Input: part model. Units: mm. Frame: model coordinates. Face numbers are marked on the shaded views. A direction names the side the tool comes from. Give positions to 0.01 mm unless a question says otherwise; leave off trailing zeros. Loops run counter-clockwise (first coordinate to the right, second up) from the corner with the lowest first, then second, coordinate; pieces in that order, holes last. Notation, with made-up numbers: (20, 50) - (52, 50) arc R13 cw to (52, 58) - close; hole circle Ø7 at (59.5, -36). An arc over 180 degrees is marked (long way). Answer as a JSON object with one key per item and string values.
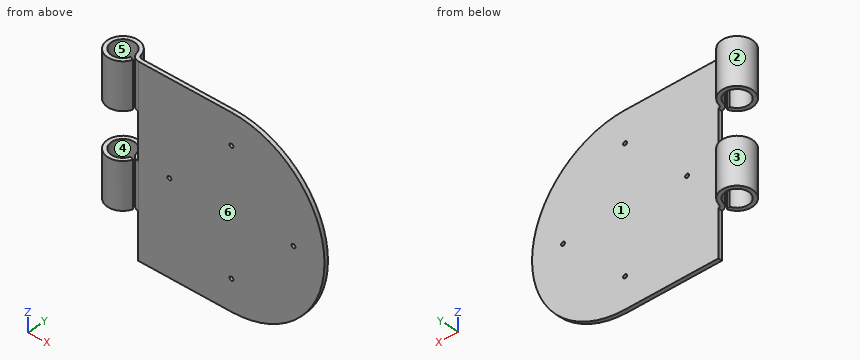
from build123d import *

# Parameters (mm, degrees)
BOSS_EXTRUDE1_DEPTH     = 76.2
CUT_EXTRUDE1_DEPTH      = 109.055004078
CUT_EXTRUDE1_DEPTH_BACK = 109.055004078
SKETCH2_W               = 19.05
SKETCH2_H               = 13.97
SKETCH3_R               = 0.79375
CUT_EXTRUDE2_DEPTH      = 114.673225775


with BuildPart() as part:
    # Sketch1 → Boss-Extrude1 (new body)
    with BuildSketch(Plane.XY):
        with BuildLine():
            Line((6.006670832, -2.059710057), (4.505003124, -1.544782543))
            ThreePointArc((4.505003124, -1.544782543), (-4.752599731, 0.306923518), (4.66627796, 0.9525))
            ThreePointArc((4.66627796, 0.9525), (5.769083619, -0.871844425), (7.777129933, -1.5875))
            Line((7.777129933, -1.5875), (83.977129933, -1.5875))
            Line((83.977129933, -1.5875), (83.977129933, 0))
            Line((83.977129933, 0), (7.777129933, 0))
            ThreePointArc((7.777129933, 0), (6.773106776, 0.357827788), (6.221703947, 1.27))
            ThreePointArc((6.221703947, 1.27), (-6.336799641, 0.409231357), (6.006670832, -2.059710057))
        make_face()
    extrude(amount=BOSS_EXTRUDE1_DEPTH)

    # Sketch2 → Cut-Extrude1 (cut, two sides: drawn at the far end of the back side and taken through both)
    with BuildSketch(Plane(origin=(69.85, -1.5875, 0), x_dir=(0, 0, -1), z_dir=(0, 1, 0)).offset(-CUT_EXTRUDE1_DEPTH_BACK)):
        with Locations((-9.525, 69.215)):
            Rectangle(SKETCH2_W, SKETCH2_H)
        with Locations((-47.625, 69.215)):
            Rectangle(SKETCH2_W, SKETCH2_H)
    extrude(amount=CUT_EXTRUDE1_DEPTH + CUT_EXTRUDE1_DEPTH_BACK, mode=Mode.SUBTRACT)

    # Sketch3 → Cut-Extrude2 (cut, through all)
    with BuildSketch(Plane(origin=(0, -1.5875, 0), x_dir=(1, 0, 0), z_dir=(0, 1, 0))):
        with BuildLine():
            Line((83.977129933, 0), (45.877129933, 0))
            ThreePointArc((45.877129933, 0), (72.817898258, -11.159231598), (83.977129933, -38.09999989))
            Line((83.977129933, -38.09999989), (83.977129933, 0))
        make_face()
        with BuildLine():
            Line((83.977129933, -76.2), (83.977129933, -38.09999989))
            ThreePointArc((83.977129933, -38.09999989), (72.817898336, -65.040768324), (45.877129933, -76.2))
            Line((45.877129933, -76.2), (83.977129933, -76.2))
        make_face()
        with Locations(Location((45.877129933, -63.5, 0), (0, 0, 90))):
            Circle(SKETCH3_R)
        with Locations(Location((20.477129933, -38.1, 0), (0, 0, 90))):
            Circle(SKETCH3_R)
        with Locations(Location((71.277129933, -38.1, 0), (0, 0, 90))):
            Circle(SKETCH3_R)
        with Locations(Location((45.877129933, -12.7, 0), (0, 0, 90))):
            Circle(SKETCH3_R)
    extrude(amount=CUT_EXTRUDE2_DEPTH, mode=Mode.SUBTRACT)


solid = part.part
Item 1: Cut plane B-B (y = 3). Return loops of the section in (x, z).
Geometry check:
{"outline": "(-5.6, 19.05) - (-3.7, 19.05) - (-3.7, 38.1) - (-5.6, 38.1) - close; (-5.6, 57.15) - (-3.7, 57.15) - (-3.7, 76.2) - (-5.6, 76.2) - close; (3.7, 19.05) - (5.6, 19.05) - (5.6, 38.1) - (3.7, 38.1) - close; (3.7, 57.15) - (5.6, 57.15) - (5.6, 76.2) - (3.7, 76.2) - close"}
Item 2: Cut plane A-A (x = 0). Return loops of the section in (y, z), then the cut area to 3 significant figures.
Geometry check:
{"outline": "(-6.35, 19.05) - (-4.76, 19.05) - (-4.76, 38.1) - (-6.35, 38.1) - close; (-6.35, 57.15) - (-4.76, 57.15) - (-4.76, 76.2) - (-6.35, 76.2) - close; (4.76, 19.05) - (6.35, 19.05) - (6.35, 38.1) - (4.76, 38.1) - close; (4.76, 57.15) - (6.35, 57.15) - (6.35, 76.2) - (4.76, 76.2) - close", "area": "121 mm2"}
Item 3: Access query for the marked faces 1 and 2. Directions: +Z, -Z, +X, -X, +Y, -Y. A direction counts if a zero-diameter tool reaches every point of the face in a straight line with its end or side. Return the directions, or none.
Geometry check:
{"face 1": "+Z, -Z, +X, +Y", "face 2": "+Z, -Z"}
Item 4: Mould query, pull axis Y, two halves, no side actions, for the marked faces 3, 4, 5 and 6. Classes: released by +Y, released by -Y, zero draft, split by the parting line, or undercut.
Geometry check:
{"face 3": "split by the parting line", "face 4": "undercut", "face 5": "undercut", "face 6": "released by -Y"}
Item 5: Material intervals for line 1 (Y direction, x = 0, z = 31.25); line 2 (X direction, y = -0.5, z = 63.5); line 3 (X direction, y = -0.75, z = 63.5), sorted ascending. Write a range as [from, to].
Geometry check:
{"line 1": "y = [-6.35, -4.76], [4.76, 6.35]", "line 2": "x = [-6.33, -4.74], [5.38, 45.08], [46.67, 74.28]", "line 3": "x = [-6.31, -4.7], [5.63, 45.08], [46.67, 74.28]"}
Item 6: Contact query for flat-ended pins moving along their axis: P1, Ø1.8, axis at x = 45.88, z = 12.7, coming from the +Y side; P2, Ø2, axis at y = -2, z = 44.5, coming from the -X side; P3, Ø1.3, axis at x = 45.88, z = 63.5, coming from the -Y side; P4, Ø1, axis at y = -1, z = 34, coming from the -X side. Output: stop coordinate, or through.
Geometry check:
{"P1": "stops at y = 0", "P2": "stops at x = 7.62", "P3": "passes through", "P4": "stops at x = -6.33"}
Item 7: Cut plane D-D (x = 51). Return loops of the section in (y, z), then the cut area to 3 significant figures.
Geometry check:
{"outline": "(-1.59, 0.35) - (0, 0.35) - (0, 75.85) - (-1.59, 75.85) - close", "area": "120 mm2"}
